Design review of the part built by this model. Coordinates are the model's own, in mm. Coordinates: 2 decimals unless noted, no trailing zeros. Loops run counter-clockwise (first coordinate to the right, second up) from the corner with the lowest first, then second, coordinate; pieces in that order, holes last. Notation, with made-up numbers: (-37.5, 8.25) -> (-31.5, 8.25) arc R27 cw to (-31.5, 24.25) -> close; hole circle Ø7 at (86, 36). An arc over 180 degrees is marked (long way). Answer as a JSON object with one key per item and string values.
Solid Edge part; units mm, degrees
sketch "Sketch1" plane through (0, 0, 0) normal (0, 0, 1) x (1, 0, 0)
  line L0 (51.9615, -30) -> (0, 60)
  line L1 (0, 60) -> (-51.9615, -30)
  line L2 (-51.9615, -30) -> (51.9615, -30)
extrude "Protrusion1" add sketch "Sketch1" along normal blind 110
sketch "Sketch2" plane through (0, 15, 110) normal (0, 0, 1) x (-0.5, 0.866, 0)
  line L0 (-64.9519, -22.5) -> (-12.9904, 67.5)
  line L1 (-12.9904, 67.5) -> (38.9711, -22.5)
  line L2 (38.9711, -22.5) -> (-64.9519, -22.5)
extrude "Cutout1" cut sketch "Sketch2" against normal up to vertex (25.1509 mm away)
sketch "Sketch3" plane through (0, 0, 0) normal (1, 0, 0) x (0, 1, 0)
  line L0 (0, 84.8491) -> (-30, 0)
extrude "ExtrudedCutout_2" cut sketch "Sketch3" along normal mid plane 220 material side at (0, -15.0471, 42.4412)
pattern_circular "Pattern1" count 3 over 360 about axis through (0, 0, 84.8491) along (0, 0, -1) of "ExtrudedCutout_2"
1) Add section B-B, the plane z = 23. Give the boundary of the cut face in (x, y), and give its area (3 significant figures).
Completed:
{"outline": "(-37.88, -21.87) -> (37.88, -21.87) -> (0, 43.74) -> close", "area": "2,480 mm²"}
2) Wall thickness on probe 1 along Z at (x, y) = (-21, 11.5); probe 2 along Y at (x, z) = (-10, 57.5); probe 3 along X at (y, z) = (34, 33.5): over which ranges is each line inside the solid? List them lowest first.
Completed:
{"probe 1": "0 to 17.15", "probe 2": "-9.67 to 2.02", "probe 3": "-1.33 to 1.33"}
3) Clearance check with flat-ended pins moving along their axes: pin 1 Ø5 at (x, z) = (15, 42) entering from +Y; pin 2 Ø1 at (y, z) = (-9.5, 39) entering from -X; pin 3 Ø6 at (y, z) = (7.5, 71.5) entering from +X. State where each tip first meets the part, or that it passes through.
Completed:
{"pin 1": "y = 9", "pin 2": "x = -24.56", "pin 3": "x = 3.24"}
